from build123d import *

# Parameters (mm, degrees)
SKETCH1_R           = 1.2192
BOSS_EXTRUDE1_DEPTH = 1.9558
SKETCH3_W           = 9.144
SKETCH3_H           = 1.016
CUT_EXTRUDE1_DEPTH  = 2.159
FILLET1_R           = 0.762
CUT_EXTRUDE2_DEPTH  = 5.7625


with BuildPart() as part:
    # Sketch1 → Boss-Extrude1 (new body)
    with BuildSketch(Plane(origin=(0, 0, 0), x_dir=(1, 0, 0), z_dir=(0, 1, 0))):
        with BuildLine():
            Line((-11.43, 2.38125), (11.43, 2.38125))
            ThreePointArc((11.43, 2.38125), (13.81125, 0), (11.43, -2.38125))
            Line((11.43, -2.38125), (-11.43, -2.38125))
            ThreePointArc((-11.43, -2.38125), (-13.81125, 0), (-11.43, 2.38125))
        make_face()
        with Locations((-11.43, 0)):
            Circle(SKETCH1_R, mode=Mode.SUBTRACT)
        with Locations((11.43, 0)):
            Circle(SKETCH1_R, mode=Mode.SUBTRACT)
    extrude(amount=BOSS_EXTRUDE1_DEPTH)

    # Sketch3 → Cut-Extrude1 (cut)
    with BuildSketch(Plane(origin=(0, 0, -2.38125), x_dir=(-1, 0, 0), z_dir=(0, 0, -1))):
        with Locations((-2.413, 1.4478)):
            Rectangle(SKETCH3_W, SKETCH3_H)
    extrude(amount=-CUT_EXTRUDE1_DEPTH, mode=Mode.SUBTRACT)

    # Fillet1
    fillet1_edges = [part.edges().sort_by_distance(p)[0] for p in [
        (6.985, 1.4478, -0.22225),
        (-2.159, 1.4478, -0.22225),
    ]]
    fillet(fillet1_edges, radius=FILLET1_R)

    # Sketch4 → Cut-Extrude2 (cut, through all)
    with BuildSketch(Plane(origin=(0, 0, -2.38125), x_dir=(-1, 0, 0), z_dir=(0, 0, -1))):
        Polygon((-8.36295, 0), (-9.04875, 0.6858), (-14.591138831, 0.6858), (-14.591138831, 0), align=None)
        Polygon((14.591138831, 0.6858), (14.591138831, 0), (8.36295, 0), (9.04875, 0.6858), align=None)
    extrude(amount=-CUT_EXTRUDE2_DEPTH, mode=Mode.SUBTRACT)


solid = part.part
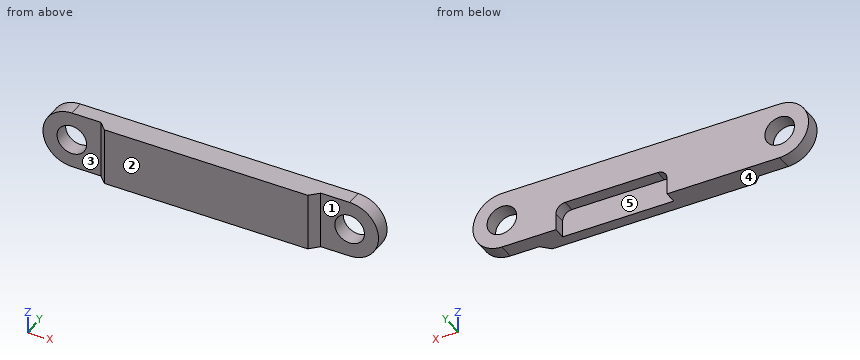
Design review of the part built by this model. Coordinates are the model's own, in mm. Face numbers are marked on the shaded views. A direction names the side the tool comes from. Coordinates: 2 decimals unless noted, no trailing zeros. Loops run counter-clockwise (first coordinate to the right, second up) from the corner with the lowest first, then second, coordinate; pieces in that order, holes last.
Item 1: Draft analysis for pull direction X (two halves, no side actions). For the marked faces 4 and 5, state which applies: pulls with the +X half, pulls with the -X half, needs draft (parallel to the pull), parting line crosses it, or undercut.
Completed:
face 4: needs draft
face 5: undercut
Item 2: For the marked faces 1, 2 and 3, list the 3-axis set-ups (+Z, -Z, +X, -X, +Y, -Y) from which the entire face can be reached by the end or side of a thin tool; tool diameter is ignored.
Completed:
face 1: +Z, -Z, +X, -Y
face 2: +Z, -Z, +X, -X, -Y
face 3: +Z, -Z, -X, -Y
Item 3: Add section D-D (x = 0.5). Write out the cut boundary in (y, z).
Completed:
outline: (0, -2.38) - (0.94, -2.38) - (0.94, -0.22) - (1.96, -0.22) - (1.96, 2.38) - (0, 2.38) - close
Item 4: Add section C-C (x = 11). Write out the cut boundary in (y, z).
Completed:
outline: (0.69, -2.38) - (1.96, -2.38) - (1.96, -1.14) - (0.69, -1.14) - close; (0.69, 1.14) - (1.96, 1.14) - (1.96, 2.38) - (0.69, 2.38) - close
Item 5: Add section A-A (y = 1.5). Write out the cut boundary in (x, z) (1 decimal), and give its area (3 significant figures).
Completed:
outline: (-11.4, -2.4) - (-2.2, -2.4) - (-2.2, -1) arc R0.8 cw to (-1.4, -0.2) - (6.2, -0.2) arc R0.8 cw to (7, -1) - (7, -2.4) - (11.4, -2.4) arc R2.4 ccw to (11.4, 2.4) - (-11.4, 2.4) arc R2.4 ccw to start; hole circle Ø2.4 at (-11.4, 0); hole circle Ø2.4 at (11.4, 0)
area: 97.9 mm2
Item 6: Add section B-B (z = 0.3). Write out the cut boundary in (x, y), and give its area (3 significant figures).
Completed:
outline: (-13.79, 0.69) - (-12.61, 0.69) - (-12.61, 1.96) - (-13.79, 1.96) - close; (-10.25, 0.69) - (-9.05, 0.69) - (-8.36, 0) - (8.36, 0) - (9.05, 0.69) - (10.25, 0.69) - (10.25, 1.96) - (-10.25, 1.96) - close; (12.61, 0.69) - (13.79, 0.69) - (13.79, 1.96) - (12.61, 1.96) - close
area: 41.0 mm2
Item 7: Clearance check with flat-ended pins moving along their axes: pin 1 (1.1 mm diameter, centred on y = 1.5, z = -1.5, fed in from +X); pin 2 (1.1 mm diameter, centred on y = 1.5, z = -1.5, fed in from -X); pin 3 (1.4 mm diameter, centred on x = -10.5, z = -0.5, fed in from -Y). State where each tip first meets the part, or that it passes through.
Completed:
pin 1: stops at x = 13.61
pin 2: stops at x = -13.61
pin 3: stops at y = 0.69
Item 8: Wall thickness on L1, parallel to X at y = 1.6, z = 0; L2, parallel to Z at x = 11.5, y = 0.8; L3, parallel to Y at x = 11.75, z = -1.5: over which ranges is each line inside the solid? List them lowest first.
Completed:
L1: x = -13.81 to -12.65, -10.21 to 10.21, 12.65 to 13.81
L2: z = -2.38 to -1.22, 1.22 to 2.38
L3: y = 0.69 to 1.96
